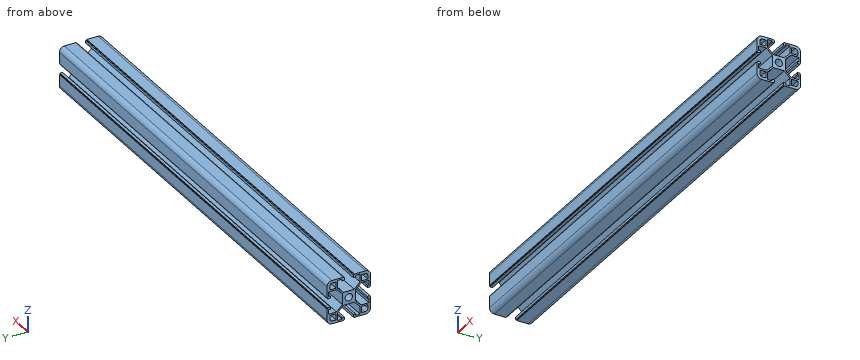
```python
from build123d import *

# Parameters (mm, degrees)
SKETCH1_R                 = 3.4
F_40_X_40L_X_R4_5_1_DEPTH = 430
SKETCH_2_R                = 2.5
CUT_EXTRUDE_1_DEPTH       = 220.60191256


with BuildPart() as part:
    # Sketch1 → 铝型材 40 X 40L X R4.5(1) (new body)
    with BuildSketch(Plane(origin=(-215, 0, 0), x_dir=(0, 0, -1), z_dir=(1, 0, 0))):
        with BuildLine():
            Line((-5.1, 20), (-5.1, 19.5))
            Line((-5.1, 19.5), (-4.1, 19.5))
            Line((-4.1, 19.5), (-4.1, 17))
            Line((-4.1, 17), (-6.1, 17))
            Line((-6.1, 17), (-6.1, 18.5))
            Line((-6.1, 18.5), (-10.3, 18.5))
            Line((-10.3, 18.5), (-10.3, 11.3))
            Line((-10.3, 11.3), (-5, 6))
            Line((-5, 6), (5, 6))
            Line((5, 6), (10.3, 11.3))
            Line((10.3, 11.3), (10.3, 18.5))
            Line((10.3, 18.5), (6.1, 18.5))
            Line((6.1, 18.5), (6.1, 17))
            Line((6.1, 17), (4.1, 17))
            Line((4.1, 17), (4.1, 19.5))
            Line((4.1, 19.5), (5.1, 19.5))
            Line((5.1, 19.5), (5.1, 20))
            Line((5.1, 20), (15.5, 20))
            ThreePointArc((15.5, 20), (18.681980515, 18.681980515), (20, 15.5))
            Line((20, 15.5), (20, 5.1))
            Line((20, 5.1), (19.5, 5.1))
            Line((19.5, 5.1), (19.5, 4.1))
            Line((19.5, 4.1), (17, 4.1))
            Line((17, 4.1), (17, 6.1))
            Line((17, 6.1), (18.5, 6.1))
            Line((18.5, 6.1), (18.5, 10.3))
            Line((18.5, 10.3), (11.3, 10.3))
            Line((11.3, 10.3), (6, 5))
            Line((6, 5), (6, -5))
            Line((6, -5), (11.3, -10.3))
            Line((11.3, -10.3), (18.5, -10.3))
            Line((18.5, -10.3), (18.5, -6.1))
            Line((18.5, -6.1), (17, -6.1))
            Line((17, -6.1), (17, -4.1))
            Line((17, -4.1), (19.5, -4.1))
            Line((19.5, -4.1), (19.5, -5.1))
            Line((19.5, -5.1), (20, -5.1))
            Line((20, -5.1), (20, -15.5))
            ThreePointArc((20, -15.5), (18.681980515, -18.681980515), (15.5, -20))
            Line((15.5, -20), (5.1, -20))
            Line((5.1, -20), (5.1, -19.5))
            Line((5.1, -19.5), (4.1, -19.5))
            Line((4.1, -19.5), (4.1, -17))
            Line((4.1, -17), (6.1, -17))
            Line((6.1, -17), (6.1, -18.5))
            Line((6.1, -18.5), (10.3, -18.5))
            Line((10.3, -18.5), (10.3, -11.3))
            Line((10.3, -11.3), (5, -6))
            Line((5, -6), (-5, -6))
            Line((-5, -6), (-10.3, -11.3))
            Line((-10.3, -11.3), (-10.3, -18.5))
            Line((-10.3, -18.5), (-6.1, -18.5))
            Line((-6.1, -18.5), (-6.1, -17))
            Line((-6.1, -17), (-4.1, -17))
            Line((-4.1, -17), (-4.1, -19.5))
            Line((-4.1, -19.5), (-5.1, -19.5))
            Line((-5.1, -19.5), (-5.1, -20))
            Line((-5.1, -20), (-15.5, -20))
            ThreePointArc((-15.5, -20), (-18.681980515, -18.681980515), (-20, -15.5))
            Line((-20, -15.5), (-20, -5.1))
            Line((-20, -5.1), (-19.5, -5.1))
            Line((-19.5, -5.1), (-19.5, -4.1))
            Line((-19.5, -4.1), (-17, -4.1))
            Line((-17, -4.1), (-17, -6.1))
            Line((-17, -6.1), (-18.5, -6.1))
            Line((-18.5, -6.1), (-18.5, -10.3))
            Line((-18.5, -10.3), (-11.3, -10.3))
            Line((-11.3, -10.3), (-6, -5))
            Line((-6, -5), (-6, 5))
            Line((-6, 5), (-11.3, 10.3))
            Line((-11.3, 10.3), (-18.5, 10.3))
            Line((-18.5, 10.3), (-18.5, 6.1))
            Line((-18.5, 6.1), (-17, 6.1))
            Line((-17, 6.1), (-17, 4.1))
            Line((-17, 4.1), (-19.5, 4.1))
            Line((-19.5, 4.1), (-19.5, 5.1))
            Line((-19.5, 5.1), (-20, 5.1))
            Line((-20, 5.1), (-20, 15.5))
            ThreePointArc((-20, 15.5), (-18.681980515, 18.681980515), (-15.5, 20))
            Line((-15.5, 20), (-5.1, 20))
        make_face()
        Circle(SKETCH1_R, mode=Mode.SUBTRACT)
        with BuildLine():
            Line((11.8, 17.5), (15, 17.5))
            ThreePointArc((15, 17.5), (16.767766953, 16.767766953), (17.5, 15))
            Line((17.5, 15), (17.5, 11.8))
            Line((17.5, 11.8), (11.8, 11.8))
            Line((11.8, 11.8), (11.8, 17.5))
        make_face(mode=Mode.SUBTRACT)
        with BuildLine():
            Line((-15, 17.5), (-11.8, 17.5))
            Line((-11.8, 17.5), (-11.8, 11.8))
            Line((-11.8, 11.8), (-17.5, 11.8))
            Line((-17.5, 11.8), (-17.5, 15))
            ThreePointArc((-17.5, 15), (-16.767766953, 16.767766953), (-15, 17.5))
        make_face(mode=Mode.SUBTRACT)
        with BuildLine():
            Line((-17.5, -11.8), (-11.8, -11.8))
            Line((-11.8, -11.8), (-11.8, -17.5))
            Line((-11.8, -17.5), (-15, -17.5))
            ThreePointArc((-15, -17.5), (-16.767766953, -16.767766953), (-17.5, -15))
            Line((-17.5, -15), (-17.5, -11.8))
        make_face(mode=Mode.SUBTRACT)
        with BuildLine():
            Line((11.8, -11.8), (17.5, -11.8))
            Line((17.5, -11.8), (17.5, -15))
            ThreePointArc((17.5, -15), (16.767766953, -16.767766953), (15, -17.5))
            Line((15, -17.5), (11.8, -17.5))
            Line((11.8, -17.5), (11.8, -11.8))
        make_face(mode=Mode.SUBTRACT)
    extrude(amount=F_40_X_40L_X_R4_5_1_DEPTH)

    # 草图2 → 切除-拉伸1 (cut, through all)
    with BuildSketch(Plane(origin=(0, 20, 0), x_dir=(1, 0, 0), z_dir=(0, 1, 0))):
        with Locations(Location((-1, 0, 0), (0, 0, 270))):
            Circle(SKETCH_2_R)
        with Locations(Location((108, 0, 0), (0, 0, 270))):
            Circle(SKETCH_2_R)
    extrude(amount=-CUT_EXTRUDE_1_DEPTH, mode=Mode.SUBTRACT)


solid = part.part
```
Build history of the part. All positions in model axes, mm. Give positions to 0.01 mm unless a question says otherwise; leave off trailing zeros. One line per question, with ' | ' between items.
Q1. Drop flat-ended pins along their axis: pin 1 (6 mm diameter, centred on y = -14, z = 2.5, fed in from -X); pin 2 (1.2 mm diameter, centred on x = -13, y = 17.5, fed in from +Z); pin 3 (4 mm diameter, centred on x = -80.5, z = 1.5, fed in from +Y). Give the stop position or say it passes through.
Filled sheet:
pin 1: passes through | pin 2: stops at z = 19.78 | pin 3: stops at y = 6
Q2. Cut at A-A, the plane x = -161. Count the separate pieces of the cut face and the enclosed holes in it, plus the area to 3 significant figures.
Filled sheet:
separate pieces: 1 | enclosed holes: 5 | area: 475 mm²
Q3. Drill centre lines: line 1 along Z through (x, y) = (-157, 15); line 2 along Z through (x, y) = (108, -4.9). Where is each one in solid material? Low to high. Write a range as [from, to].
Filled sheet:
line 1: z = [-20, -17.5], [-11.8, -10.3], [10.3, 11.8], [17.5, 20] | line 2: z = [-19.5, -17], [-6, -2.5], [2.5, 6], [17, 19.5]
